Verification items for the finished model (mm, model axes). Face numbers are marked on the shaded views. A direction names the side the tool comes from. Round coordinates to 2 decimals unless told otherwise and drop trailing zeros. Write each loop counter-clockwise with the first axis right and the second up, starting at its lowest first coordinate (ties: lowest second). Pieces come first, ordered by that corner, then holes. Notation, with made-up numbers: M 78.25,-37 L 99.25,-37 A26 cw 99.25,-15 Z; hole C 66.25,70.25 d4. An arc over 180 degrees is marked long. One line per question, with ' | ' between items.
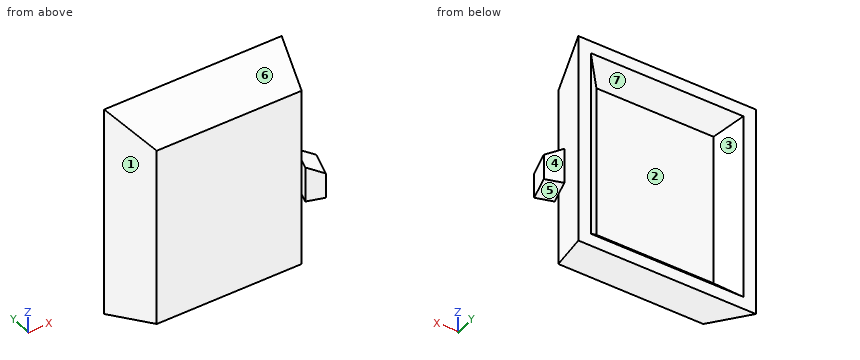
from build123d import *

# Parameters (mm, degrees)
SKETCH1_W           = 100
SKETCH1_H           = 120
BOSS_EXTRUDE1_DEPTH = 30
BOSS_EXTRUDE1_DRAFT = -17
SKETCH2_W           = 86
SKETCH2_H           = 106
CUT_EXTRUDE1_DEPTH  = 10
SKETCH3_W           = 20
SKETCH3_H           = 15
BOSS_EXTRUDE2_DEPTH = 10
DRAFT1_ANGLE        = 45
DRAFT2_ANGLE        = 30


with BuildPart() as part:
    # Sketch1 → Boss-Extrude1 (with draft: the straight prism first)
    with BuildSketch(Plane(origin=(0, 0, 0), x_dir=(1, 0, 0), z_dir=(0, 1, 0))):
        Rectangle(SKETCH1_W, SKETCH1_H)
    extrude(amount=-BOSS_EXTRUDE1_DEPTH)
    # Boss-Extrude1: the draft: its side faces are tilted about the plane it starts from
    boss_extrude1_sides = [part.faces().sort_by_distance(p)[0] for p in [
        (-50, -15, 0),
        (0, -15, 60),
        (50, -15, 0),
        (0, -15, -60),
    ]]
    draft(boss_extrude1_sides, Plane(origin=(0, 0, 0), x_dir=(1, 0, 0), z_dir=(0, 1, 0)), BOSS_EXTRUDE1_DRAFT)

    # Sketch2 → Cut-Extrude1 (cut)
    with BuildSketch(Plane(origin=(0, 0, 0), x_dir=(1, 0, 0), z_dir=(0, 1, 0))):
        Rectangle(SKETCH2_W, SKETCH2_H)
    extrude(amount=-CUT_EXTRUDE1_DEPTH, mode=Mode.SUBTRACT)

    # Sketch3 → Boss-Extrude2 (add)
    with BuildSketch(Plane(origin=(45.725939314, -13.979822587, 0), x_dir=(0, 0, -1), z_dir=(0.9563047559630354, -0.2923717047227369, 0))):
        with Locations((0, -15)):
            Rectangle(SKETCH3_W, SKETCH3_H)
    extrude(amount=BOSS_EXTRUDE2_DEPTH)

    # Draft1
    draft1_faces = [part.faces().sort_by_distance(p)[0] for p in [
        (0, -5, 53),
        (43, -5, 0),
        (0, -5, -53),
        (-43, -5, 0),
    ]]
    draft(draft1_faces, Plane.ZX, DRAFT1_ANGLE)

    # Draft2
    draft2_faces = [part.faces().sort_by_distance(p)[0] for p in [
        (46.121887523, -29.78625245, 10),
    ]]
    draft(draft2_faces, Plane(origin=(50, 0, -60), x_dir=(0.2923717047227369, 0.9563047559630354, 0), z_dir=(0.9563047559630354, -0.2923717047227369, 0)), DRAFT2_ANGLE)


solid = part.part
1. Section check C-C, the plane y = -8.5. Record the cut outline in (x, z).
Results:
outline: M -47.4,-57.4 L 47.4,-57.4 L 47.4,57.4 L -47.4,57.4 Z; hole M -34.5,-44.5 L 34.5,-44.5 L 34.5,44.5 L -34.5,44.5 Z
2. Section check A-A, the plane x = 30. Record the cut outline in (y, z).
Results:
outline: M -30,-50.83 L 0,-60 L 0,-53 L -10,-43 L -10,43 L 0,53 L 0,60 L -30,50.83 Z
3. Section check D-D, the plane y = -2.5. Record the cut outline in (x, z).
Results:
outline: M -49.24,-59.24 L 49.24,-59.24 L 49.24,59.24 L -49.24,59.24 Z; hole M -40.5,-50.5 L 40.5,-50.5 L 40.5,50.5 L -40.5,50.5 Z
4. Mould release check, pull along X, two halves, no side actions. Record for the marked faces 1, 2, 3 and 4: pulls with the +X half, pulls with the -X half, needs draft (parallel to the pull), parting line crosses it, or undercut.
Results:
face 1: pulls with the -X half | face 2: undercut | face 3: undercut | face 4: pulls with the +X half
5. Tool access check on the marked faces 5, 6 and 7. Record the directions out of +Z, -Z, +X, -X, +Y, -Y that give a thin tool (end or side, any length) a straight path to the whole face; none if there is none.
Results:
face 5: -Z, +X, -Y | face 6: +Z, +X, -X, -Y | face 7: +Y
6. Thickness scan on line 1 (Y direction, x = -25.5, z = 12); line 2 (X direction, y = -23, z = 29); line 3 (Z direction, x = 32.5, y = -3.5). Record the ranges inside material, lowest first.
Results:
line 1: y = -30 to -10 | line 2: x = -42.97 to 42.97 | line 3: z = -58.93 to -49.5, 49.5 to 58.93
7. Go/stop test with flat-tipped pins: P1, Ø1, axis at x = -25, y = -22.5, coming from the +Z side; P2, Ø12, axis at x = 13, z = -1, coming from the -Y side; P3, Ø4, axis at x = 33, z = -33, coming from the +Y side. Record where each tip stops, or that it passes through.
Results:
P1: stops at z = 53.27 | P2: stops at y = -30 | P3: stops at y = -8
8. Section check B-B, the plane z = 47.5. Record the cut outline in (x, y), then the cut area to 3 significant figures.
Results:
outline: M -50,0 L -40.83,-30 L 40.83,-30 L 50,0 L 43,0 L 37.5,-5.5 L -37.5,-5.5 L -43,0 Z | area: 2,280 mm2
